from build123d import *

# Parameters (mm, degrees)
SKETCH2_R               = 4
CUT_EXTRUDE1_DEPTH      = 58.350893629
CUT_EXTRUDE2_DEPTH      = 58.350893629
CUT_EXTRUDE2_DEPTH_BACK = 1
SKETCH3_R               = 6.5


with BuildPart() as part:
    # Sketch1 → Revolve1 (revolve)
    with BuildSketch(Plane.XY, mode=Mode.PRIVATE) as revolve1_sk:
        Polygon((0, 0), (0, 4), (-22.991533214, 4), (-28.865230633, -3), (-40.25, -3), (-40.25, -7), (-27, -7), (-21.126302582, 0), align=None)
    revolve(revolve1_sk.sketch.rotate(Axis((0, 4, 0), (0, -1, 0)), 270), axis=Axis((0, 4, 0), (0, -1, 0)))

    # Sketch2 → Cut-Extrude1 (cut, through all)
    with BuildSketch(Plane(origin=(0, -3, 0), x_dir=(1, 0, 0), z_dir=(0, 1, 0))):
        with Locations(Location((0, 32, 0), (0, 0, 270))):
            Circle(SKETCH2_R)
        with Locations(Location((27.712812921, -16, 0), (0, 0, 270))):
            Circle(SKETCH2_R)
        with Locations(Location((-27.712812921, -16, 0), (0, 0, 270))):
            Circle(SKETCH2_R)
    extrude(amount=-CUT_EXTRUDE1_DEPTH, mode=Mode.SUBTRACT)

    # Sketch3 → Cut-Extrude2 (cut, two sides: drawn at the far end of the back side and taken through both)
    with BuildSketch(Plane(origin=(0, -3, 0), x_dir=(1, 0, 0), z_dir=(0, 1, 0)).offset(-CUT_EXTRUDE2_DEPTH_BACK)):
        with Locations(Location((0, 32, 0), (0, 0, 325.92949513))):
            Circle(SKETCH3_R)
        with Locations(Location((27.712812921, -16, 0), (0, 0, 94.070504949))):
            Circle(SKETCH3_R)
        with Locations(Location((-27.712812921, -16, 0), (0, 0, 85.92949513))):
            Circle(SKETCH3_R)
    extrude(amount=CUT_EXTRUDE2_DEPTH + CUT_EXTRUDE2_DEPTH_BACK, mode=Mode.SUBTRACT)


solid = part.part
Input: part model. Units: mm. Frame: model coordinates. A direction names the side the tool comes from. Coordinates: 2 decimals unless noted, no trailing zeros. Order: outer loops, then holes, each group sorted by start corner. A loop starts at its lowest first (then second) coordinate and runs counter-clockwise, first axis right, second up. Notation, with made-up numbers: M -22,12 L 21,12 A29 ccw 21,32 Z; hole C -22,29 d1. An arc over 180 degrees is marked long. Write item = value, one per line. Start each with the question number.
(1) Section D-D on z = 16. Give the number of separate pieces and of enclosed holes in the cut face, and give its area (3 significant figures).
(2) First-contact query: P1, Ø10.5, axis at x = -27.71, z = 16, coming from the +Y side; P2, Ø1.5, axis at x = 10.5, y = -5, coming from the -Z side; P3, Ø10.5, axis at x = 30.5, z = 19, coming from the +Y side. Flat tips, straight axial feed; report the tip coordinate or a pass-through.
(3) Pull-direction query (X, two-part tool) for faces 1 (the cylindrical face through (30.416, -5.479, 13.052)), 2 (the flat face through (0, 4, 0)), 3 (the flat face through (-2.5, -4, -28.5)), 4 (the conical face through (-23.16, 3.56, -3.04)); classes: released by +X, released by -X, zero draft, split by the parting line, or undercut.
(4) Line query: line 1 along Y through (x, z) = (-23.5, 26.5); line 2 along Z through (x, y) = (-14.5, -0.5); line 3 along X through (y, z) = (-5.75, -8.5). Output: solid intervals per line, ascending. Write a range as [from, to].
(5) Section B-B on z = 0. Output: boundary loops of the cut face in (x, y).
(6) Section C-C on y = -6. Output: boundary loops of the cut face in (x, z).
(7) Section A-A on z = -32. Output: boundary loops of the cut face in (x, y), and give its area (3 significant figures).
(8) Reachability of faces 5 (the flat face through (-18, -3, -24)), 6 (the cylindrical face through (-12.09, -5.03, 38.39)), 7 (the flat face through (0, 0, 0)) from +Z, -Z, +X, -X, +Y, -Y: full face, straight path, thin tool, end or side. Return the list, or none.
Result set:
q1.separate_pieces = 3
q1.enclosed_holes = 0
q1.area = 248 mm²
q2.P1 = -4
q2.P2 = -39.05
q2.P3 = -3
q3.face_1 = undercut
q3.face_2 = zero draft
q3.face_3 = undercut
q3.face_4 = split by the parting line
q4.line_1 = [-7, -3]
q4.line_2 = [-22.5, -15.94], [15.94, 22.5]
q4.line_3 = [-39.34, -24.52], [24.52, 39.34]
q5.outline = M -40.25,-7 L -27,-7 L -21.13,0 L 21.13,0 L 27,-7 L 40.25,-7 L 40.25,-3 L 28.87,-3 L 22.99,4 L -22.99,4 L -28.87,-3 L -40.25,-3 Z
q6.outline = C 0,0 d80.5; hole C -27.71,16 d8; hole C 0,0 d52.32; hole C 0,-32 d8; hole C 27.71,16 d8
q7.outline = M -24.41,-7 L -4,-7 L -4,-4 L -6.5,-4 L -6.5,-3 L -24.41,-3 Z; M 4,-7 L 24.41,-7 L 24.41,-3 L 6.5,-3 L 6.5,-4 L 4,-4 Z
q7.area = 158 mm²
q8.face_5 = +Y
q8.face_6 = +Y, -Y
q8.face_7 = -Y
